For this review, use the dimensioned drawing (mm, ordinates from the lowest corner) and the shaded views. Round coordinates to 2 decimals unless told otherwise and drop trailing zeros. Write each loop counter-clockwise with the first axis right and the second up, starting at its lowest first coordinate (ties: lowest second). Pieces come first, ordered by that corner, then holes. Notation, with made-up numbers: M 13.25,23.25 L 49.25,23.25 A17 ccw 49.25,52.25 Z; hole C 8.25,13 d4. An arc over 180 degrees is marked long. Use one line per item in the form item = value. Start each with the question number.
Item 1: Add section A-A (z = 119). State the section outline as (x, y) points.
Item 2: For P1, Ø1.8, axis at x = 38, z = 134.5, coming from the -Y side; P2, Ø11.5, axis at x = 22.5, z = 13.25, coming from the +Y side; P3, Ø1.9, axis at y = 1.5, z = 56.5, coming from the -X side; P4, Ø1.5, axis at x = 6, y = 3, coming from the -Z side, all flat-tipped, find the tip position at first contact; note any pin that passes through.
Item 3: For line 1 (X direction, y = 3.5, z = 134.5); line 2 (Z direction, x = 22.5, y = 4.75); line 3 (Z direction, x = 7, y = 1.75), list the stretches that pass through material, from the lowest coordinate up. Write a range as [from, to].
Item 4: Add section C-C (x = 22.5). State the section outline as (y, z) points.
Item 5: Add section B-B (z = 103.5). State the section outline as (x, y) points, and give its area (3 significant figures).
Item 6: Add section D-D (y = 4.75). State the section outline as (x, z) points, and give its area (3 significant figures).
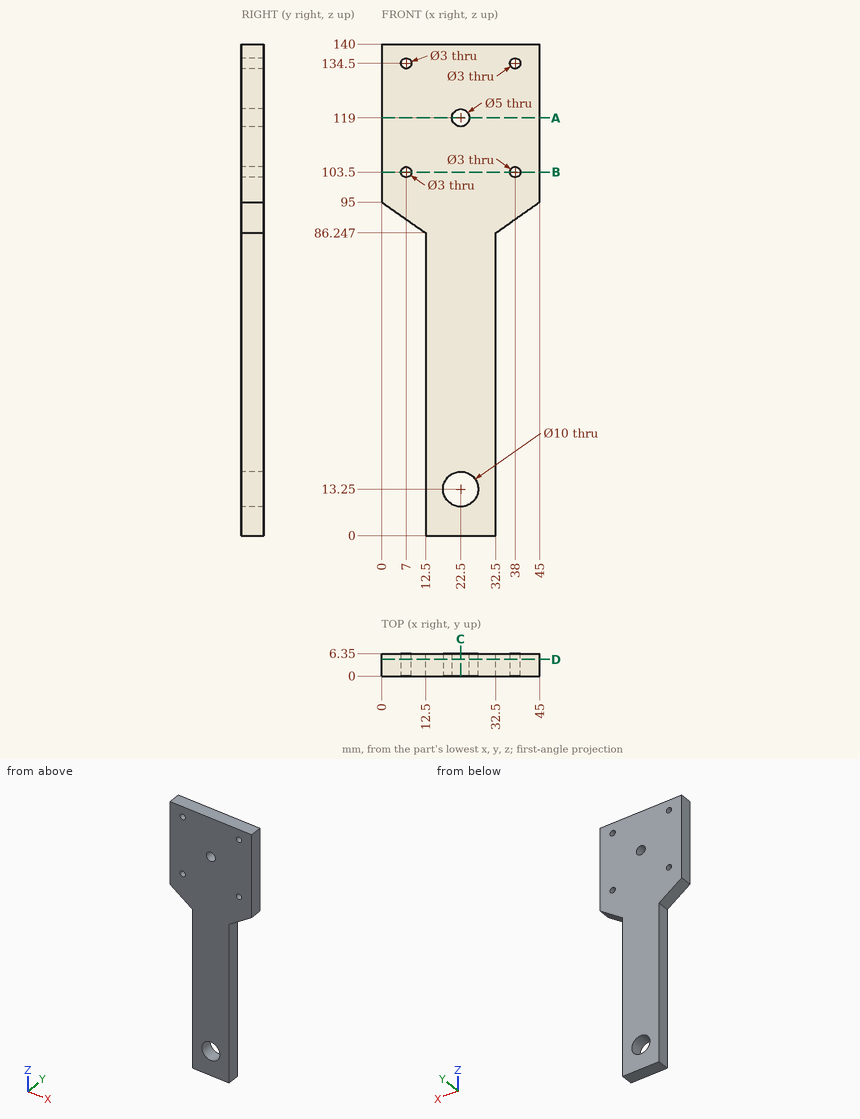
Calculated:
q1.outline = M 0,0 L 20,0 L 20,6.35 L 0,6.35 Z; M 25,0 L 45,0 L 45,6.35 L 25,6.35 Z
q2.P1 = through
q2.P2 = 6.35
q2.P3 = 12.5
q2.P4 = 90.27
q3.line_1 = [0, 5.5], [8.5, 36.5], [39.5, 45]
q3.line_2 = [0, 8.25], [18.25, 116.5], [121.5, 140]
q3.line_3 = [90.1, 102], [105, 133], [136, 140]
q4.outline = M 0,0 L 6.35,0 L 6.35,8.25 L 0,8.25 Z; M 0,18.25 L 6.35,18.25 L 6.35,116.5 L 0,116.5 Z; M 0,121.5 L 6.35,121.5 L 6.35,140 L 0,140 Z
q5.outline = M 0,0 L 5.5,0 L 5.5,6.35 L 0,6.35 Z; M 8.5,0 L 36.5,0 L 36.5,6.35 L 8.5,6.35 Z; M 39.5,0 L 45,0 L 45,6.35 L 39.5,6.35 Z
q5.area = 248 mm^2
q6.outline = M 0,95 L 12.5,86.25 L 12.5,0 L 32.5,0 L 32.5,86.25 L 45,95 L 45,140 L 0,140 Z; hole C 7,103.5 d3; hole C 7,134.5 d3; hole C 22.5,13.25 d10; hole C 22.5,119 d5; hole C 38,103.5 d3; hole C 38,134.5 d3
q6.area = 3,910 mm^2
